from build123d import *

# Parameters (mm, degrees)
F1_DEPTH = 25.4


with BuildPart() as f1:
    # F0 (on Right) → F1 (new body)
    with BuildSketch(Plane.YZ):
        with BuildLine():
            ThreePointArc((9.525, 50.8), (6.7351920908, 44.0648079092), (0, 41.275))
            Line((0, 41.275), (0, 15.875))
            ThreePointArc((0, 15.875), (10.5003255055, 11.9062500091), (15.7504882702, 1.9843750273))
            Line((15.7504882702, 1.9843750273), (9.4502929642, 51.990625))
            ThreePointArc((9.4502929642, 51.990625), (9.5063048942, 51.396483242), (9.525, 50.8))
        make_face()
        with BuildLine():
            Line((0, 15.875), (0, 41.275))
            ThreePointArc((0, 41.275), (-7.14375, 44.4998046905), (-9.4502929642, 51.990625))
            Line((-9.4502929642, 51.990625), (-15.7504883051, 1.9843747505))
            ThreePointArc((-15.7504883051, 1.9843747505), (-10.5003256101, 11.9062499168), (0, 15.875))
        make_face()
        with BuildLine():
            ThreePointArc((-9.4502929642, 51.990625), (-7.14375, 44.4998046905), (0, 41.275))
            ThreePointArc((0, 41.275), (6.7351920908, 44.0648079092), (9.525, 50.8))
            ThreePointArc((9.525, 50.8), (9.5063048942, 51.396483242), (9.4502929642, 51.990625))
            ThreePointArc((9.4502929642, 51.990625), (0, 60.325), (-9.4502929642, 51.990625))
        make_face()
        with BuildLine():
            ThreePointArc((15.7504882702, 1.9843750273), (10.5003255055, 11.9062500091), (0, 15.875))
            Line((0, 15.875), (0, -15.875))
            ThreePointArc((0, -15.875), (10.5003255381, -11.9062499803), (15.7504882811, -1.984374941))
            ThreePointArc((15.7504882811, -1.984374941), (15.8438414922, -0.994138707), (15.875, 0))
            ThreePointArc((15.875, 0), (15.8438414895, 0.9941387503), (15.7504882702, 1.9843750273))
        make_face()
        with BuildLine():
            Line((0, -15.875), (0, 15.875))
            ThreePointArc((0, 15.875), (-10.5003256101, 11.9062499168), (-15.7504883051, 1.9843747505))
            ThreePointArc((-15.7504883051, 1.9843747505), (-11.9062499168, -10.5003256101), (0, -15.875))
        make_face()
        with BuildLine():
            ThreePointArc((15.7504882811, -1.984374941), (10.5003255381, -11.9062499803), (0, -15.875))
            Line((0, -15.875), (0, -53.975))
            ThreePointArc((0, -53.975), (6.7351920908, -56.7648079092), (9.525, -63.5))
            Line((9.525, -63.5), (36.5125, -63.5))
            ThreePointArc((36.5125, -63.5), (38.9384772185, -57.7879930953), (44.7334821429, -55.5675637964))
            Line((44.7334821429, -55.5675637964), (17.8507837718, -54.6068545332))
            ThreePointArc((17.8507837718, -54.6068545332), (12.0791026517, -51.812957818), (10.2468749586, -45.6679514317))
            Line((10.2468749586, -45.6679514317), (15.7504882811, -1.984374941))
        make_face()
        with BuildLine():
            Line((0, -53.975), (0, -15.875))
            ThreePointArc((0, -15.875), (-11.9062499168, -10.5003256101), (-15.7504883051, 1.9843747505))
            Line((-15.7504883051, 1.9843747505), (-16.0004960241, 0))
            Line((-16.0004960241, 0), (-9.525, -63.5))
            ThreePointArc((-9.525, -63.5), (-6.7351920908, -56.7648079092), (0, -53.975))
        make_face()
        with BuildLine():
            Line((16.0004960241, 0), (15.7504882702, 1.9843750273))
            ThreePointArc((15.7504882702, 1.9843750273), (15.8438414895, 0.9941387503), (15.875, 0))
            ThreePointArc((15.875, 0), (15.8438414922, -0.994138707), (15.7504882811, -1.984374941))
            Line((15.7504882811, -1.984374941), (16.0004960241, 0))
        make_face()
        with BuildLine():
            Line((0, -63.5), (0, -53.975))
            ThreePointArc((0, -53.975), (-6.7351920908, -56.7648079092), (-9.525, -63.5))
            ThreePointArc((-9.525, -63.5), (-6.7351920908, -70.2351920908), (0, -73.025))
            Line((0, -73.025), (0.6773435479, -73.000885786))
            ThreePointArc((0.6773435479, -73.000885786), (6.9705567315, -69.9912990883), (9.525, -63.5))
            Line((9.525, -63.5), (0, -63.5))
        make_face()
        with BuildLine():
            Line((36.5125, -63.5), (9.525, -63.5))
            ThreePointArc((9.525, -63.5), (6.9705567315, -69.9912990883), (0.6773435479, -73.000885786))
            Line((0.6773435479, -73.000885786), (44.7324052746, -71.4324746146))
            ThreePointArc((44.7324052746, -71.4324746146), (38.9380895153, -69.2116327839), (36.5125, -63.5))
        make_face()
        with BuildLine():
            ThreePointArc((44.7334821429, -55.5675637964), (38.9384772185, -57.7879930953), (36.5125, -63.5))
            ThreePointArc((36.5125, -63.5), (38.9380895153, -69.2116327839), (44.7324052746, -71.4324746146))
            ThreePointArc((44.7324052746, -71.4324746146), (50.1616327839, -69.0119104847), (52.3875, -63.5))
            ThreePointArc((52.3875, -63.5), (50.1620069047, -57.9884772185), (44.7334821429, -55.5675637964))
        make_face()
        with BuildLine():
            ThreePointArc((0, -73.025), (0.3388863295, -73.0189695375), (0.6773435479, -73.000885786))
            Line((0.6773435479, -73.000885786), (0, -73.025))
        make_face()
    extrude(amount=F1_DEPTH)


solid = f1.part
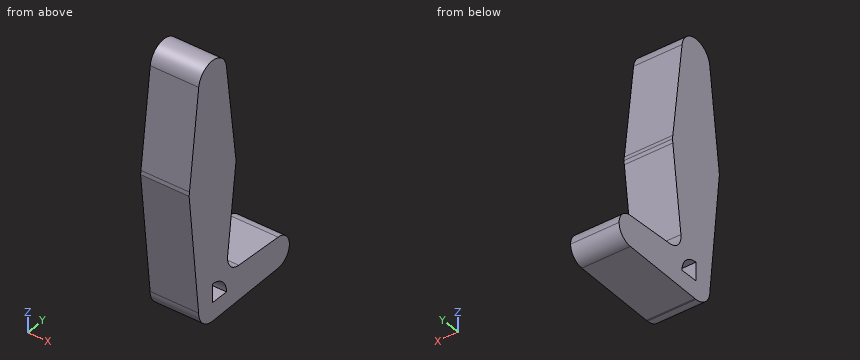
Verification items for the finished model (mm, model axes). Coordinates: 2 decimals unless noted, no trailing zeros. Order: outer loops, then holes, each group sorted by start corner. A loop starts at its lowest first (then second) coordinate and runs counter-clockwise, first axis right, second up. Notation, with made-up numbers: M 64,29 L 77,29 A25 cw 77,59 Z; hole C -24.5,68 d1. An arc over 180 degrees is marked long. Write each question's results on one line, items separated by ' | '.
1) Section check B-B on y = 25. Record the cut outline in (x, z).
Solved:
outline: M 0,-72.13 L 25.4,-72.13 L 25.4,-54.86 L 0,-54.86 Z
2) Gauge pin test, flat ends, axial feed: pin 1 Ø3 at (x, z) = (21, -38) entering from +Y; pin 2 Ø2 at (x, z) = (11.5, -51.5) entering from -Y; pin 3 Ø3 at (x, y) = (12, 4) entering from +Z. Record the tip position at first contact, or that the pin passes through.
Solved:
pin 1: stops at y = 11.4 | pin 2: stops at y = -10.85 | pin 3: stops at z = 59.99
3) Scan lines: line 1 along Z through (x, y) = (15.5, 0.5); line 2 along Z through (x, y) = (14, 45); line 3 along Y through (x, z) = (5.5, 51.5). Record each from-to range of solid material in increasing order. Write a range as [from, to].
Solved:
line 1: z = [-73.01, -63.5], [-53.99, 60.31] | line 2: z = [-71.42, -55.58] | line 3: y = [-9.51, 9.51]
4) Section check C-C on z = 18. Record the cut outline in (x, y).
Solved:
outline: M 0,-13.73 L 25.4,-13.73 L 25.4,13.73 L 0,13.73 Z
